from build123d import *

# Parameters (mm, degrees)
F1_DEPTH = 812.8
F2_R     = 6.35
F2_R_2   = 3.175
F3_DEPTH = 25.4
F4_R     = 3.175
F5_DEPTH = 25.4


with BuildPart() as f1:
    # F0 (on Front) → F1 (new body)
    with BuildSketch(Plane.XZ):
        Polygon((0, -3.175), (0, 0), (0, 34.925), (-3.175, 34.925), (-3.175, -3.175), align=None)
    extrude(amount=F1_DEPTH)

    # F2 (on face) → F3 (cut)
    with BuildSketch(Plane.YZ):
        with Locations((-330.2, 15.875)):
            Circle(F2_R)
        with Locations((-346.71, 5.715)):
            Circle(F2_R_2)
        with Locations((-313.69, 5.715)):
            Circle(F2_R_2)
    extrude(amount=-F3_DEPTH, mode=Mode.SUBTRACT)

    # F4 (on face) → F5 (cut)
    with BuildSketch(Plane.YZ):
        with Locations((-20.366231, 15.875)):
            Circle(F4_R)
        with Locations((-141.016231, 15.875)):
            Circle(F4_R)
        with Locations((-261.666231, 15.875)):
            Circle(F4_R)
        with Locations((-382.316231, 15.875)):
            Circle(F4_R)
        with Locations((-502.966231, 15.875)):
            Circle(F4_R)
        with Locations((-623.616231, 15.875)):
            Circle(F4_R)
        with Locations((-744.266231, 15.875)):
            Circle(F4_R)
    extrude(amount=-F5_DEPTH, mode=Mode.SUBTRACT)


solid = f1.part
The listing builds one solid part. Answer for the finished solid, in the listing's coordinates (mm). Give positions to 0.01 mm unless a question says otherwise; leave off trailing zeros. Answer as a JSON object with one key per item and string values.
1. A flat-ended cylindrical pin translates along its axis: pin 1 Ø5 at (y, z) = (-313.69, 5.715) entering from -X. Find the tip coordinate at first contact, or state that the pin passes through.
Determined:
{"pin 1": "through"}
2. Find the intervals of material crossed by L1, parallel to Y at x = -0.25, z = 6; L2, parallel to Z at x = -0.7, y = -382 (3 decimals); L3, parallel to Z at x = -1.3, y = -346.71 (3 decimals), in increasing order. Write a range as [from, to].
Determined:
{"L1": "[-812.8, -349.87], [-343.55, -316.85], [-310.53, 0]", "L2": "[-3.175, 12.716], [19.034, 34.925]", "L3": "[-3.175, 2.54], [8.89, 34.925]"}
3. For a pull along Z with two mould halves and no side action, classify faces 1 (the flat face through (0, -401, 16)), 2 (the cylindrical face through (-1.565, -324.334, 13.443)) as pulls with the +Z half, pulls with the -Z half, needs draft (parallel to the pull), parting line crosses it, or undercut.
Determined:
{"face 1": "needs draft", "face 2": "undercut"}
